Autodesk Fusion 360 part; units mm, degrees
sketch "Sketch1" plane through (0, 0, 0) normal (0, 0, 1) x (1, 0, 0)
  line L0 (0, 0) -> (60, 0)
  line L1 (60, 0) -> (60, 25)
  line L2 (60, 25) -> (0, 25)
  line L3 (0, 25) -> (0, 0)
  line L4 (5, 20) -> (55, 20)
  line L5 (55, 20) -> (55, 5)
  line L6 (55, 5) -> (5, 5)
  line L7 (5, 5) -> (5, 20)
  line L8 (10.5, 16) -> (17.5, 16)
  line L9 (17.5, 16) -> (17.5, 9)
  line L10 (17.5, 9) -> (10.5, 9)
  line L11 (10.5, 9) -> (10.5, 16)
  line L12 (42.5, 16) -> (49.5, 16)
  line L13 (49.5, 16) -> (49.5, 9)
  line L14 (49.5, 9) -> (42.5, 9)
  line L15 (42.5, 9) -> (42.5, 16)
  dimension "d1" = 60
  dimension "d2" = 25
  dimension "d3" = 50
  dimension "d4" = 15
  dimension "d5" = 5
  dimension "d7" = 5
  dimension "d8" = 7
  dimension "d9" = 7
  dimension "d10" = 4
  dimension "d12" = 7
  dimension "d13" = 7
  dimension "d15" = 4
  dimension "d16" = 5.5
  dimension "d17" = 5.5
  dimension "d18" = 25
sketch "Sketch2" plane through (0, 0, 0) normal (0, 0, 1) x (1, 0, 0)
extrude "Extrude1" add sketch "Sketch1" along normal blind 3 contours L0 L1 L2 L3 | L4 L5 L6 L7
sketch "Sketch3" plane through (0, 0, 0) normal (0, -1, 0) x (1, 0, 0)
  line L0 (0, 0) -> (60, 0)
  line L1 (60, 0) -> (60, 3)
  line L2 (60, 3) -> (0, 3)
  line L3 (0, 3) -> (0, 0)
  line L4 (25, 2) -> (35, 2)
  line L5 (35, 2) -> (35, 0)
  line L6 (35, 0) -> (25, 0)
  line L7 (25, 0) -> (25, 2)
  dimension "d21" = 10
extrude "Extrude2" add sketch "Sketch3" along normal blind 30 contours L0 L4 L5 L6 L7
sketch "Sketch4" plane through (0, 25, 0) normal (0, 1, 0) x (-1, 0, 0)
  line L0 (-60, 0) -> (0, 0)
  line L1 (0, 0) -> (0, 3)
  line L2 (0, 3) -> (-60, 3)
  line L3 (-60, 3) -> (-60, 0)
  line L4 (-35, 2) -> (-25, 2)
  line L5 (-25, 2) -> (-25, 0)
  line L6 (-25, 0) -> (-35, 0)
  line L7 (-35, 0) -> (-35, 2)
extrude "Extrude3" add sketch "Sketch4" along normal blind 30 contours L0 L4 L5 L6 L7
sketch "Sketch5" plane through (35, 0, 0) normal (1, 0, 0) x (0, 1, 0)
  line L0 (25, 2) -> (25, 0)
  line L1 (25, 0) -> (55, 0)
  line L2 (55, 0) -> (55, 2)
  line L3 (55, 2) -> (25, 2)
  line L4 (50, 1) -> (55, 1)
  line L5 (55, 1) -> (55, 0)
  line L6 (55, 0) -> (50, 0)
  line L7 (50, 0) -> (50, 1)
extrude "Extrude4" add sketch "Sketch5" along normal blind 30 contours L1 L2 L4 L5 L6 L7
sketch "Sketch6" plane through (25, 0, 0) normal (-1, 0, 0) x (0, -1, 0)
  line L0 (-25, 0) -> (-25, 2)
  line L1 (-25, 2) -> (-55, 2)
  line L2 (-55, 2) -> (-55, 0)
  line L3 (-55, 0) -> (-25, 0)
  line L4 (-50, 1) -> (-55, 1)
  line L5 (-55, 1) -> (-55, 0)
  line L6 (-55, 0) -> (-50, 0)
  line L7 (-50, 0) -> (-50, 1)
extrude "Extrude5" add sketch "Sketch6" along normal blind 30 contours L2 L3 L4 L5 L6 L7
sketch "Sketch7" plane through (35, 0, 0) normal (1, 0, 0) x (0, 1, 0)
  line L0 (0, 0) -> (0, 2)
  line L1 (0, 2) -> (-30, 2)
  line L2 (-30, 2) -> (-30, 0)
  line L3 (-30, 0) -> (0, 0)
  line L4 (-30, 2) -> (-25, 2)
  line L5 (-25, 2) -> (-25, 0)
  line L6 (-25, 0) -> (-30, 0)
  line L7 (-30, 0) -> (-30, 2)
extrude "Extrude6" add sketch "Sketch7" along normal blind 30 contours L1 L2 L3 L4 L5 L6 L7
sketch "Sketch8" plane through (25, 0, 0) normal (-1, 0, 0) x (0, -1, 0)
  line L0 (0, 2) -> (0, 0)
  line L1 (0, 0) -> (30, 0)
  line L2 (30, 0) -> (30, 2)
  line L3 (30, 2) -> (0, 2)
  line L4 (25, 2) -> (30, 2)
  line L5 (30, 2) -> (30, 0)
  line L6 (30, 0) -> (25, 0)
  line L7 (25, 0) -> (25, 2)
extrude "Extrude7" add sketch "Sketch8" along normal blind 30 contours L1 L2 L3 L4 L5 L6 L7
Read the model definition and answer for the solid it produces. Units are mm, in the model's axes. A direction names the side the tool comes from. Coordinates: 2 decimals unless noted, no trailing zeros. Write each loop counter-clockwise with the first axis right and the second up, starting at its lowest first coordinate (ties: lowest second). Pieces come first, ordered by that corner, then holes. Notation, with made-up numbers: (-7.5, -31) -> (35.5, -31) arc R16 ccw to (35.5, -14) -> close; hole circle Ø3 at (46.5, 24). An arc over 180 degrees is marked (long way). Return JSON: item names as keys, results as strings.
(1) For a pull along Y with two mould halves and no side action, classify faces 4 (the flat face through (30, -30, 1)), 5 (the flat face through (35, 40, 1)), 6 (the flat face through (-5, -27, 1)) as pulls with the +Y half, pulls with the -Y half, needs draft (parallel to the pull), parting line crosses it, or undercut.
Answers below:
{"face 4": "pulls with the -Y half", "face 5": "undercut", "face 6": "needs draft"}
(2) Each of these flat-tipped pins is pushed along its axis until it touches: P1, Ø3, axis at x = 37.5, y = -5, coming from the +Z side; P2, Ø0.9, axis at y = 8, z = 1.5, coming from the +X side; P3, Ø1.5, axis at y = 11.5, z = 2, coming from the -X side; P4, Ø4, axis at x = 53, y = 52, coming from the +Z side. Where does it stop, or does it pass through?
Answers below:
{"P1": "through", "P2": "x = 60", "P3": "x = 0", "P4": "z = 1"}
(3) The part is cut by section A-A on x = 51.5. Give the vertices of the cut face in (y, z), then the cut area to 3 significant figures.
Answers below:
{"outline": "(-30, 0) -> (-25, 0) -> (-25, 2) -> (-30, 2) -> close; (0, 0) -> (25, 0) -> (25, 3) -> (0, 3) -> close; (50, 0) -> (55, 0) -> (55, 1) -> (50, 1) -> close", "area": "90.0 mm^2"}
(4) The part is cut by section C-C on y = 46.5. Give the vertices of the cut face in (x, z).
Answers below:
{"outline": "(25, 0) -> (35, 0) -> (35, 2) -> (25, 2) -> close"}
(5) The part is cut by section D-D on y = 5. Give the vertices of the cut face in (x, z).
Answers below:
{"outline": "(0, 0) -> (60, 0) -> (60, 3) -> (0, 3) -> close"}
(6) Which of the six approach directions +Z, -Z, +X, -X, +Y, -Y give full straight-line access (tool end or side, diameter ignored) to faces 1 (the flat face through (33, -22, 2)), 2 (the flat face through (50, -25, 1)), 3 (the flat face through (10.5, 12, 1))?
Answers below:
{"face 1": "+Z, +X, -X, -Y", "face 2": "+Z, -Z, +X", "face 3": "+Z, -Z"}
(7) The part is cut by section B-B on x = 61.5. Give the vertices of the cut face in (y, z), then the cut area to 3 significant figures.
Answers below:
{"outline": "(-30, 0) -> (-25, 0) -> (-25, 2) -> (-30, 2) -> close; (50, 0) -> (55, 0) -> (55, 1) -> (50, 1) -> close", "area": "15.0 mm^2"}
(8) Consider line 1 along X through (y, z) = (11.5, 1); line 2 along Y through (x, z) = (39, 0.85); line 3 along Y through (x, z) = (7.5, 1.7). Determine where each line is inside the solid, lowest interval first. Write a range as from..to.
Answers below:
{"line 1": "0..10.5, 17.5..42.5, 49.5..60", "line 2": "-30..-25, 0..25, 50..55", "line 3": "-30..-25, 0..25"}
